Geometry check sheet. Reference: drawing and pictorial views, mm from the part's lowest x, y, z. A direction names the side the tool comes from. Coordinates: 2 decimals unless noted, no trailing zeros. Write each loop counter-clockwise with the first axis right and the second up, starting at its lowest first coordinate (ties: lowest second). Pieces come first, ordered by that corner, then holes.
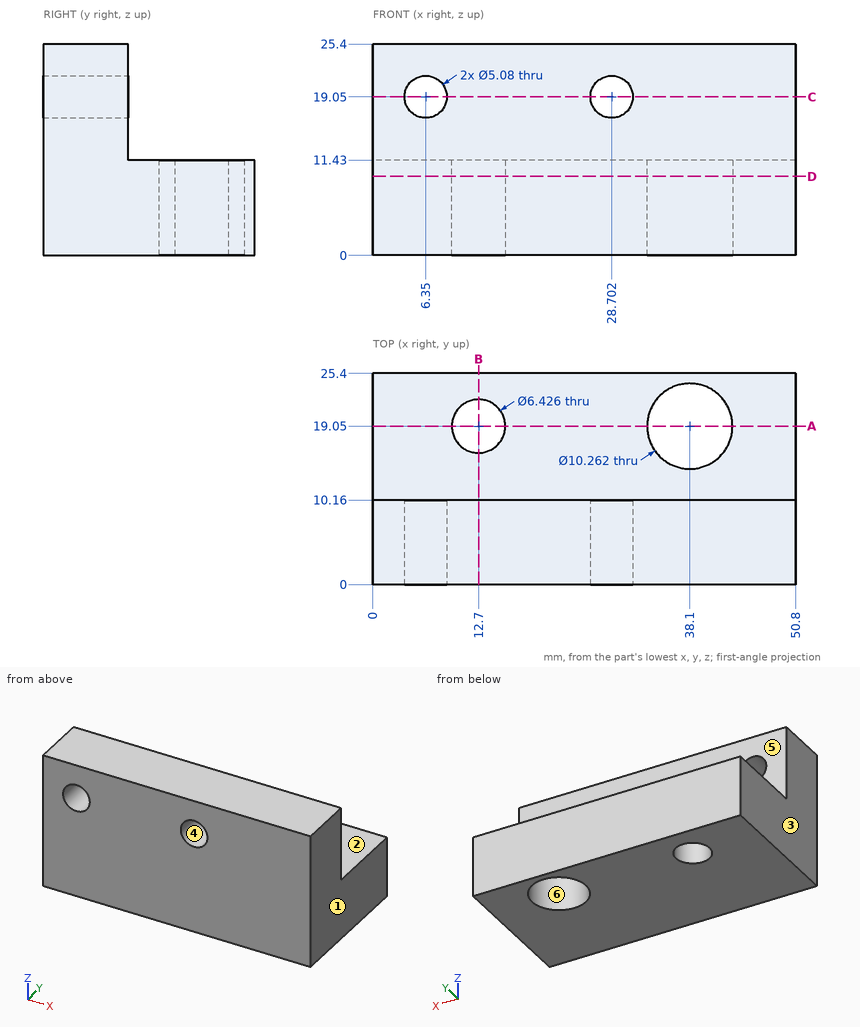
1. Sectioned sample at D-D, the plane z = 9.5. Record the boundary of the cut face in (x, y), and give its area (3 significant figures).
2. Material ranges on L1, parallel to X at y = 5.5, z = 19.05; L2, parallel to Y at x = 12.7, z = 4.5; L3, parallel to Z at x = 6.35, y = 6.25, recorded low to high.
3. Draft check along X on the marked faces 1, 2, 3 and 4. Enter one of: pulls with the +X half, pulls with the -X half, needs draft (parallel to the pull), parting line crosses it, or undercut.
4. Tool access check on the marked faces 5 and 6. Record the directions out of +Z, -Z, +X, -X, +Y, -Y that give a thin tool (end or side, any length) a straight path to the whole face; none if there is none.
5. Sectioned sample at C-C, the plane z = 19.05. Record the boundary of the cut face in (x, y), and give its area (3 significant figures).
6. Sectioned sample at A-A, the plane y = 19.05. Record the boundary of the cut face in (x, z), and give its area (3 significant figures).
7. Sectioned sample at B-B, the plane x = 12.7. Record the boundary of the cut face in (y, z).
8. Gauge pin test, flat ends, axial feed: P1, Ø6, axis at x = 8, z = 17.5, coming from the +Y side; P2, Ø12, axis at x = 16.5, y = 18.5, coming from the +Z side. Record the tip position at first contact, or that the pin passes through.
Outcome:
1. outline: (0, 0) - (50.8, 0) - (50.8, 25.4) - (0, 25.4) - close; hole circle Ø6.43 at (12.7, 19.05); hole circle Ø10.26 at (38.1, 19.05)
1. area: 1,180 mm2
2. L1: x = 0 to 3.81, 8.89 to 26.16, 31.24 to 50.8
2. L2: y = 0 to 15.84, 22.26 to 25.4
2. L3: z = 0 to 16.51, 21.59 to 25.4
3. face 1: pulls with the +X half
3. face 2: needs draft
3. face 3: pulls with the -X half
3. face 4: undercut
4. face 5: +Z, +X, -X, +Y
4. face 6: +Z, -Z
5. outline: (0, 0) - (3.81, 0) - (3.81, 10.16) - (0, 10.16) - close; (8.89, 0) - (26.16, 0) - (26.16, 10.16) - (8.89, 10.16) - close; (31.24, 0) - (50.8, 0) - (50.8, 10.16) - (31.24, 10.16) - close
5. area: 413 mm2
6. outline: (0, 0) - (9.49, 0) - (9.49, 11.43) - (0, 11.43) - close; (15.91, 0) - (32.97, 0) - (32.97, 11.43) - (15.91, 11.43) - close; (43.23, 0) - (50.8, 0) - (50.8, 11.43) - (43.23, 11.43) - close
6. area: 390 mm2
7. outline: (0, 0) - (15.84, 0) - (15.84, 11.43) - (10.16, 11.43) - (10.16, 25.4) - (0, 25.4) - close; (22.26, 0) - (25.4, 0) - (25.4, 11.43) - (22.26, 11.43) - close
8. P1: stops at y = 10.16
8. P2: stops at z = 11.43
